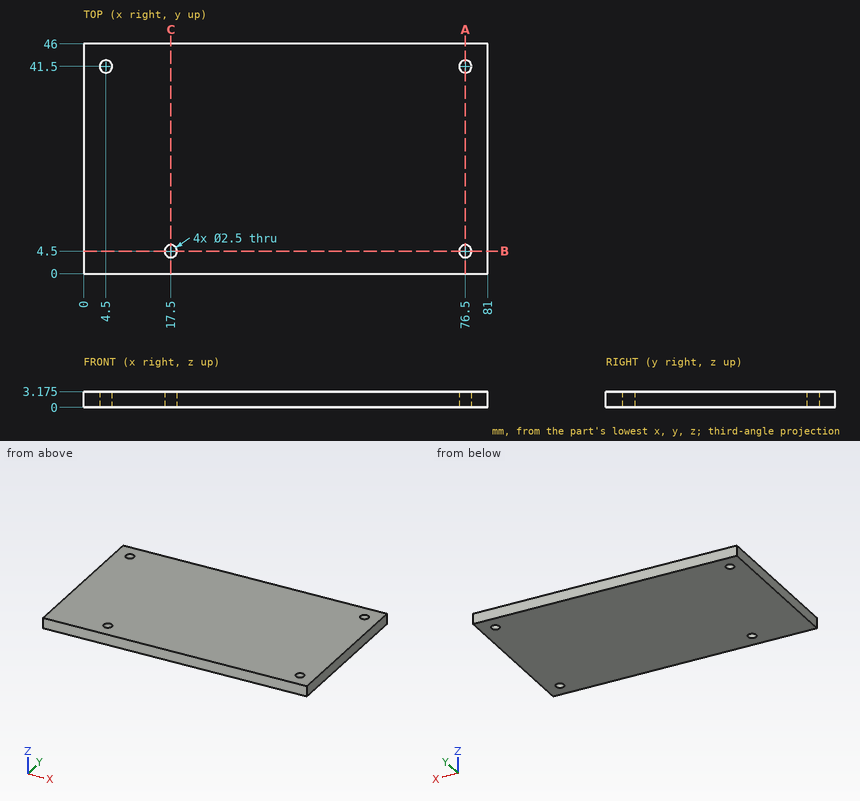
Part print with two shaded views. Sizes in mm from the minimum x, y, z corner. Give positions to 0.01 mm unless a question says otherwise; leave off trailing zeros. Order: outer loops, then holes, each group sorted by start corner. A loop starts at its lowest first (then second) coordinate and runs counter-clockwise, first axis right, second up.
1) Wall check: probe 1 along Y at (x, z) = (76.5, 1.35); probe 2 along Y at (x, z) = (17, 2.75). Give the ranges that are in metal, low to high.
2) Saw through at B-B, the plane y = 4.5. Write the cut outline in (x, z) (3 decimals).
3) Saw through at C-C, the plane x = 17.5. Write the cut outline in (y, z) (3 decimals).
4) Pin check, flat tips, straight feed: pin 1 (3 mm diameter, centred on x = 4.5, y = 41.5, fed in from -Z); pin 2 (1.5 mm diameter, centred on x = 76.5, y = 41.5, fed in from -Z). Stop position of each tip, or through.
5) Saw through at A-A, the plane x = 76.5. Write the cut outline in (y, z) (3 decimals).
Computed:
1. probe 1: y = 0 to 3.25, 5.75 to 40.25, 42.75 to 46
1. probe 2: y = 0 to 3.35, 5.65 to 46
2. outline: (0, 0) - (16.25, 0) - (16.25, 3.175) - (0, 3.175) - close; (18.75, 0) - (75.25, 0) - (75.25, 3.175) - (18.75, 3.175) - close; (77.75, 0) - (81, 0) - (81, 3.175) - (77.75, 3.175) - close
3. outline: (0, 0) - (3.25, 0) - (3.25, 3.175) - (0, 3.175) - close; (5.75, 0) - (46, 0) - (46, 3.175) - (5.75, 3.175) - close
4. pin 1: stops at z = 0
4. pin 2: passes through
5. outline: (0, 0) - (3.25, 0) - (3.25, 3.175) - (0, 3.175) - close; (5.75, 0) - (40.25, 0) - (40.25, 3.175) - (5.75, 3.175) - close; (42.75, 0) - (46, 0) - (46, 3.175) - (42.75, 3.175) - close
